Drawing for the job (mm, zero at the part's lowest x, y, z). A direction names the side the tool comes from. Give positions to 0.01 mm unless a question says otherwise; leave off trailing zeros. Write each loop counter-clockwise with the first axis right and the second up, starting at its lowest first coordinate (ties: lowest second). Pieces come first, ordered by that corner, then holes. Notation, with made-up numbers: M -30.75,12 L -5.75,12 A18 cw -5.75,18 Z; hole C 88.25,-19.75 d9. An arc over 180 degrees is marked long. Answer as a JSON object with one key per item and string values. Group by question number.
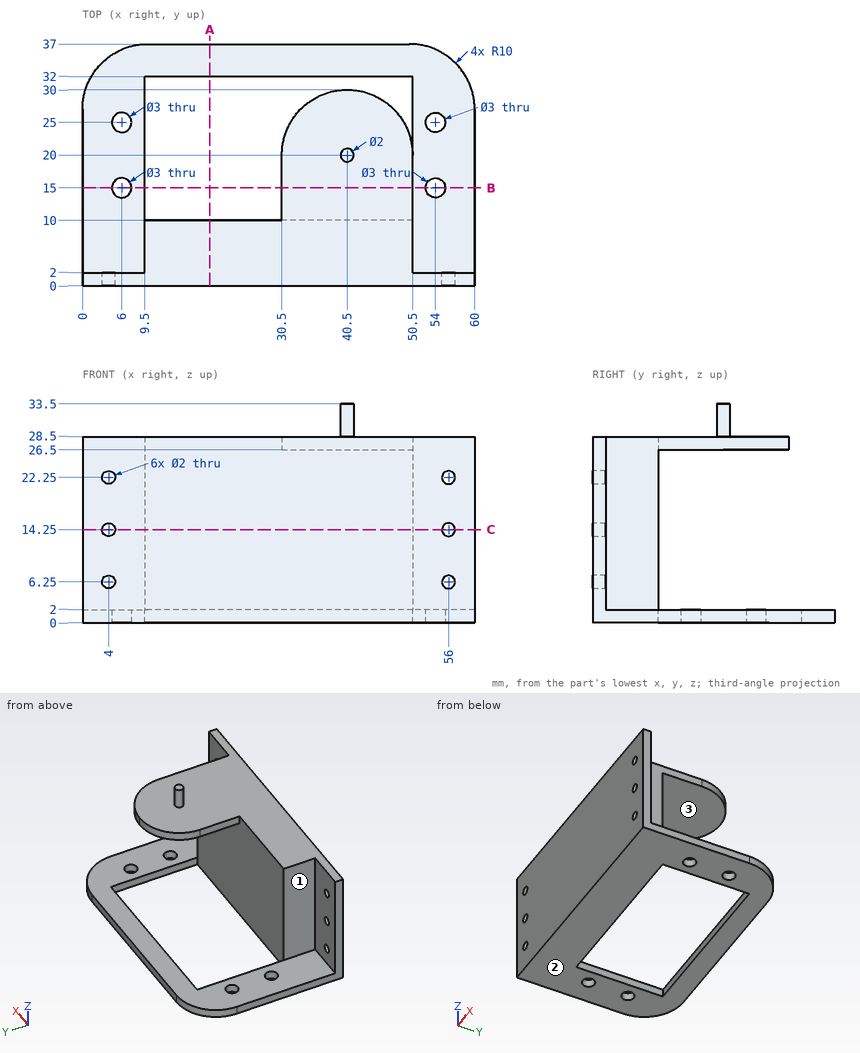
Q1. Drop flat-ended pins along their axis: P1, Ø12, axis at y = 19, z = 21, coming from the +X side; P2, Ø10, axis at x = 42.5, y = 23.5, coming from the -Z side; P3, Ø1.8, axis at x = 56, z = 6.25, coming from the -Y side; P4, Ø1, axis at y = 5.5, z = 13, coming from the -X side. Give the stop position or say it passes through.
Q2. Slice it at B-B, the plane y = 15. Write the cut outline in (x, z), then the cut area to 3 significant figures.
Q3. 3-axis set-ups, long thin cutter, end or side, ignore diameter. For the marked faces 1, 2 and 3: which of +Z, -Z, +X, -X, +Y, -Y reach the whole face in a straight line?
Q4. Slice it at C-C, the plane z = 14.25. Write the cut outline in (x, y), then the cut area to 3 significant figures.
Q5. Slice it at A-A, the plane x = 19.5. Write the cut outline in (y, z), then the cut area to 3 significant figures.
Q6. Wall check: L1, parallel to Z at x = 4, y = 1.5; L2, parallel to X at y = 1.15, z = 22.25; L3, parallel to Y at x = 54, z = 0.75 (1 decimal). Give the ranges that are in metal, low to high.
Solved:
{
 "1": {"P1": "stops at x = 50.5", "P2": "stops at z = 26.5", "P3": "passes through", "P4": "stops at x = 9.5"},
 "2": {"outline": "M 0,0 L 4.5,0 L 4.5,2 L 0,2 Z; M 7.5,0 L 9.5,0 L 9.5,2 L 7.5,2 Z; M 30.5,26.5 L 50.5,26.5 L 50.5,28.5 L 30.5,28.5 Z; M 50.5,0 L 52.5,0 L 52.5,2 L 50.5,2 Z; M 55.5,0 L 60,0 L 60,2 L 55.5,2 Z", "area": "66.0 mm²"},
 "3": {"face 1": "+Z, -X, +Y", "face 2": "-Z, +X, -X, +Y, -Y", "face 3": "-Z, +X, -X, +Y"},
 "4": {"outline": "M 0,0 L 3,0 L 3,2 L 0,2 Z; M 5,0 L 55,0 L 55,2 L 50.5,2 L 50.5,10 L 9.5,10 L 9.5,2 L 5,2 Z; M 57,0 L 60,0 L 60,2 L 57,2 Z", "area": "440 mm²"},
 "5": {"outline": "M 0,0 L 10,0 L 10,28.5 L 0,28.5 Z; M 32,0 L 37,0 L 37,2 L 32,2 Z", "area": "295 mm²"},
 "6": {"L1": "z = 0 to 5.25, 7.25 to 13.25, 15.25 to 21.25, 23.25 to 28.5", "L2": "x = 0 to 3, 5 to 55, 57 to 60", "L3": "y = 0 to 13.5, 16.5 to 23.5, 26.5 to 36.2"}
}
